```python
from build123d import *

# Parameters (mm, degrees)
DODANIE_WYCI_GNI_CIE1_DEPTH = 10
SZKIC2_R                    = 2.1
WYTNIJ_WYCI_GNI_CIE1_DEPTH  = 4
SZKIC3_R                    = 2.1
WYTNIJ_WYCI_GNI_CIE2_DEPTH  = 4
SFAZOWANIE1_SIZE            = 6
SZKIC4_W                    = 10
SZKIC4_H                    = 10
WYTNIJ_WYCI_GNI_CIE3_DEPTH  = 4
ZAOKR_GLENIE1_R             = 4


with BuildPart() as part:
    # Szkic1 → Dodanie-wyciągnięcie1 (new body)
    with BuildSketch(Plane(origin=(0, 0, 0), x_dir=(1, 0, 0), z_dir=(0, 1, 0))):
        Polygon((0, 0), (0, 150), (-20, 150), (-20, 145), (-40, 145), (-40, 140), (-10, 140), (-10, 0), align=None)
    extrude(amount=DODANIE_WYCI_GNI_CIE1_DEPTH)

    # Szkic2 → Wytnij-wyciągnięcie1 (cut)
    with BuildSketch(Plane.XZ):
        with Locations(Location((-7.2, -123, 0), (0, 0, 270))):
            Circle(SZKIC2_R)
        with Locations(Location((-7.2, -27, 0), (0, 0, 270))):
            Circle(SZKIC2_R)
    extrude(amount=-WYTNIJ_WYCI_GNI_CIE1_DEPTH, mode=Mode.SUBTRACT)

    # Szkic3 → Wytnij-wyciągnięcie2 (cut)
    with BuildSketch(Plane.XY):
        with Locations((-6, 4)):
            Circle(SZKIC3_R)
    extrude(amount=-WYTNIJ_WYCI_GNI_CIE2_DEPTH, mode=Mode.SUBTRACT)

    # Sfazowanie1
    sfazowanie1_edges = [part.edges().sort_by_distance(p)[0] for p in [
        (0, 10, -75),
    ]]
    chamfer(sfazowanie1_edges, length=SFAZOWANIE1_SIZE)

    # Szkic4 → Wytnij-wyciągnięcie3 (cut)
    with BuildSketch(Plane.XZ):
        with Locations((-5, -75)):
            Rectangle(SZKIC4_W, SZKIC4_H)
    extrude(amount=-WYTNIJ_WYCI_GNI_CIE3_DEPTH, mode=Mode.SUBTRACT)

    # Zaokrąglenie1
    zaokr_glenie1_edges = [part.edges().sort_by_distance(p)[0] for p in [
        (-5, 4, -80),
        (-5, 4, -70),
    ]]
    fillet(zaokr_glenie1_edges, radius=ZAOKR_GLENIE1_R - 0.0001)  # a hair under: the kernel refuses the full size


solid = part.part
```
Model file for the job. Use its own axes, mm. A direction names the side the tool comes from. Coordinates: 2 decimals unless noted, no trailing zeros. Write each loop counter-clockwise with the first axis right and the second up, starting at its lowest first coordinate (ties: lowest second). Pieces come first, ordered by that corner, then holes. Notation, with made-up numbers: (-18, 22.25) - (-12, 22.25) arc R21 ccw to (-12, 61.25) - close; hole circle Ø3 at (-30, -40). An arc over 180 degrees is marked (long way). Use a Markdown table: item, result. Add a question column.
Item 1: Two-plate mould, pull along X, no slides. Class faces 6 (the face through (-10, 5, -71)), 7 (the face through (-8, 1.97, -124.94)), 8 (the face through (-25, 5, -140)): pulls with the +X half, pulls with the -X half, needs draft (parallel to the pull), parting line crosses it, or undercut.
Item 2: Band-saw the part on B-B, the plane x = -34. Write the cut outline in (y, z).
Item 3: Band-saw the part on C-C, the plane z = -123. Write the cut outline in (x, y).
Item 4: Band-saw the part on D-D, the plane x = -18. Write the cut outline in (y, z), and give its area (3 significant figures).
Item 5: Drill centre lines: line 1 along X through (y, z) = (1.45, -123); line 2 along Y through (x, z) = (-6, -1.8); line 3 along Z through (x, y) = (-35, 7.5). Where is each one in solid material? Low to high.
Item 6: 3-axis set-ups, long thin cutter, end or side, ignore diameter. For faces 1 (the face through (-7, 4, -123)), 2 (the face through (-4.93, 2.797, -71.141)), 3 (the face through (-6.46, 1.95, -1.97)), 4 (the face through (-20, 5, -148)), 5 (the face through (-9.7, 0, -125.5)): which of +Z, -Z, +X, -X, +Y, -Y reach the whole face in a straight line?
Item 7: Band-saw the part on A-A, the plane z = -91. Write the cut outline in (x, y), and give its area (3 significant figures).
Item 8: Drop flat-ended pins along their axis: pin 1 (1.6 mm diameter, centred on x = -7, z = -75, fed in from -Y); pin 2 (5.5 mm diameter, centred on x = -6, y = 4, fed in from +Z); pin 3 (5 mm diameter, centred on y = 4, z = -75.5, fed in from -X); pin 4 (2 mm diameter, centred on x = -31, y = 6, fed in from +Z). Give the stop position or say it passes through.
A:
| question | item | result |
|---|---|---|
| 1 | face 6 | pulls with the -X half |
| 1 | face 7 | undercut |
| 1 | face 8 | needs draft |
| 2 | outline | (0, -145) - (10, -145) - (10, -140) - (0, -140) - close |
| 3 | outline | (-10, 0) - (-9.3, 0) - (-9.3, 4) - (-5.1, 4) - (-5.1, 0) - (0, 0) - (0, 4) - (-6, 10) - (-10, 10) - close |
| 4 | outline | (0, -150) - (10, -150) - (10, -140) - (0, -140) - close |
| 4 | area | 100 mm² |
| 5 | line 1 | x = -10 to -9.3, -5.1 to 0 |
| 5 | line 2 | y = 0 to 1.9, 6.1 to 10 |
| 5 | line 3 | z = -145 to -140 |
| 6 | face 1 | -Y |
| 6 | face 2 | +X, -X, -Y |
| 6 | face 3 | +Z |
| 6 | face 4 | -Z, -X, +Y, -Y |
| 6 | face 5 | +Z, -Z, +X, -X, -Y |
| 7 | outline | (-10, 0) - (0, 0) - (0, 4) - (-6, 10) - (-10, 10) - close |
| 7 | area | 82.0 mm² |
| 8 | pin 1 | stops at y = 4 |
| 8 | pin 2 | stops at z = 0 |
| 8 | pin 3 | stops at x = -10 |
| 8 | pin 4 | stops at z = -140 |
